Geometry check sheet. Reference: the model listing, model coordinates, mm. A direction names the side the tool comes from. Give positions to 0.01 mm unless a question says otherwise; leave off trailing zeros. Loops run counter-clockwise (first coordinate to the right, second up) from the corner with the lowest first, then second, coordinate; pieces in that order, holes last. Notation, with made-up numbers: (72.5, 32) -> (106.5, 32) arc R26 ccw to (106.5, 70) -> close; hole circle Ø8 at (0.25, 38). An arc over 180 degrees is marked (long way). Answer in a Markdown table with one row per item. Add a question column.
```python
from build123d import *

# Parameters (mm, degrees)
CROQUIS1_W               = 72
CROQUIS1_H               = 74
SALIENTE_EXTRUIR3_DEPTH  = 4
CROQUIS2_W               = 3
CROQUIS2_H               = 6
SALIENTE_EXTRUIR4_DEPTH  = 7.6
CORTAR_EXTRUIR3_DEPTH    = 83.938591741
CROQUIS5_W               = 5
CROQUIS5_H               = 4
SALIENTE_EXTRUIR5_DEPTH  = 1
CROQUIS9_W               = 72
CROQUIS9_H               = 1.5
SALIENTE_EXTRUIR6_DEPTH  = 8
CROQUIS10_W              = 72
CROQUIS10_H              = 5.9
SALIENTE_EXTRUIR7_DEPTH  = 2
CROQUIS11_W              = 10
CROQUIS11_H              = 4.4
SALIENTE_EXTRUIR10_DEPTH = 7
SALIENTE_EXTRUIR14_DEPTH = 10
CROQUIS15_W              = 18
CROQUIS15_H              = 4.4
SALIENTE_EXTRUIR15_DEPTH = 5
CROQUIS16_W              = 72
CROQUIS16_H              = 40
SALIENTE_EXTRUIR16_DEPTH = 10.5
CROQUIS17_W              = 72
CROQUIS17_H              = 5
SALIENTE_EXTRUIR17_DEPTH = 8
CROQUIS18_W              = 72
CROQUIS18_H              = 8
SALIENTE_EXTRUIR19_DEPTH = 2
CROQUIS19_W              = 72
CROQUIS19_H              = 1
CORTAR_EXTRUIR4_DEPTH    = 14.5
CROQUIS20_W              = 72
CROQUIS20_H              = 7
SALIENTE_EXTRUIR20_DEPTH = 65
CROQUIS21_W              = 57
CROQUIS21_H              = 46
CORTAR_EXTRUIR5_DEPTH    = 65


with BuildPart() as part:
    # Croquis1 → Saliente-Extruir3 (new body)
    with BuildSketch(Plane.XY):
        with Locations((0, -2.5)):
            Rectangle(CROQUIS1_W, CROQUIS1_H)
    extrude(amount=SALIENTE_EXTRUIR3_DEPTH)

    # Croquis2 → Saliente-Extruir4 (add)
    with BuildSketch(Plane.XY.offset(4)):
        with Locations((-34.5, -36.5)):
            Rectangle(CROQUIS2_W, CROQUIS2_H)
        with Locations((34.5, -36.5)):
            Rectangle(CROQUIS2_W, CROQUIS2_H)
    extrude(amount=SALIENTE_EXTRUIR4_DEPTH)

    # Croquis3 → Cortar-Extruir3 (cut, through all)
    with BuildSketch(Plane.ZY.offset(36)):
        Polygon((4, -39.5), (11.6, -36.5), (11.6, -39.5), align=None)
    extrude(amount=-CORTAR_EXTRUIR3_DEPTH, mode=Mode.SUBTRACT)

    # Croquis5 → Saliente-Extruir5 (add)
    with BuildSketch(Plane.XY.offset(4)):
        with Locations((-33.5, -30.5)):
            Rectangle(CROQUIS5_W, CROQUIS5_H)
        with Locations((33.5, -29.5)):
            Rectangle(CROQUIS5_W, CROQUIS5_H)
    extrude(amount=SALIENTE_EXTRUIR5_DEPTH)

    # Croquis9 → Saliente-Extruir6 (add)
    with BuildSketch(Plane.XY.offset(4)):
        with Locations((0, -26.35)):
            Rectangle(CROQUIS9_W, CROQUIS9_H)
    extrude(amount=SALIENTE_EXTRUIR6_DEPTH)

    # Croquis10 → Saliente-Extruir7 (add)
    with BuildSketch(Plane.XY.offset(12)):
        with Locations((0, -28.55)):
            Rectangle(CROQUIS10_W, CROQUIS10_H)
    extrude(amount=SALIENTE_EXTRUIR7_DEPTH)

    # Croquis11 → Saliente-Extruir10 (add)
    with BuildSketch(Plane.XY.offset(14)):
        with Locations((-31, -29.3)):
            Rectangle(CROQUIS11_W, CROQUIS11_H)
        with Locations((31, -29.3)):
            Rectangle(CROQUIS11_W, CROQUIS11_H)
    extrude(amount=-SALIENTE_EXTRUIR10_DEPTH)

    # Croquis14 → Saliente-Extruir14 (add)
    with BuildSketch(Plane.XY.offset(4)):
        with BuildLine():
            Line((-9, -23.7), (-9, -25.6))
            Line((-9, -25.6), (-2.1, -25.6))
            ThreePointArc((-2.1, -25.6), (-2.656497116, -24.256497116), (-4, -23.7))
            Line((-4, -23.7), (-9, -23.7))
        make_face()
        with BuildLine():
            Line((-9, -21.2), (-9, -22.2))
            Line((-9, -22.2), (-4, -22.2))
            ThreePointArc((-4, -22.2), (-2.22447191, -22.714955647), (-1, -24.1))
            Line((-1, -24.1), (1, -24.1))
            ThreePointArc((1, -24.1), (2.22447191, -22.714955647), (4, -22.2))
            Line((4, -22.2), (9, -22.2))
            Line((9, -22.2), (9, -21.2))
            Line((9, -21.2), (-9, -21.2))
        make_face()
        with BuildLine():
            ThreePointArc((4, -23.7), (2.656497116, -24.256497116), (2.1, -25.6))
            Line((2.1, -25.6), (9, -25.6))
            Line((9, -25.6), (9, -23.7))
            Line((9, -23.7), (4, -23.7))
        make_face()
    extrude(amount=SALIENTE_EXTRUIR14_DEPTH)

    # Croquis15 → Saliente-Extruir15 (add)
    with BuildSketch(Plane.XY.offset(4)):
        with Locations((0, -23.4)):
            Rectangle(CROQUIS15_W, CROQUIS15_H)
    extrude(amount=SALIENTE_EXTRUIR15_DEPTH)

    # Croquis16 → Saliente-Extruir16 (add)
    with BuildSketch(Plane.XY.offset(4)):
        with Locations((0, 14.5)):
            Rectangle(CROQUIS16_W, CROQUIS16_H)
    extrude(amount=SALIENTE_EXTRUIR16_DEPTH)

    # Croquis17 → Saliente-Extruir17 (add)
    with BuildSketch(Plane.XY.offset(14.5)):
        with Locations((0, 32)):
            Rectangle(CROQUIS17_W, CROQUIS17_H)
    extrude(amount=SALIENTE_EXTRUIR17_DEPTH)

    # Croquis18 → Saliente-Extruir19 (add)
    with BuildSketch(Plane(origin=(0, 34.5, 0), x_dir=(1, 0, 0), z_dir=(0, 1, 0))):
        with Locations((0, -18.5)):
            Rectangle(CROQUIS18_W, CROQUIS18_H)
    extrude(amount=SALIENTE_EXTRUIR19_DEPTH)

    # Croquis19 → Cortar-Extruir4 (cut)
    with BuildSketch(Plane(origin=(0, 0, 0), x_dir=(-1, 0, 0), z_dir=(0, 0, -1))):
        with Locations((0, 34)):
            Rectangle(CROQUIS19_W, CROQUIS19_H)
    extrude(amount=-CORTAR_EXTRUIR4_DEPTH, mode=Mode.SUBTRACT)

    # Croquis20 → Saliente-Extruir20 (add)
    with BuildSketch(Plane(origin=(0, 0, 0), x_dir=(-1, 0, 0), z_dir=(0, 0, -1))):
        with Locations((0, -36)):
            Rectangle(CROQUIS20_W, CROQUIS20_H)
    extrude(amount=SALIENTE_EXTRUIR20_DEPTH)

    # Croquis21 → Cortar-Extruir5 (cut)
    with BuildSketch(Plane(origin=(0, -32.5, 0), x_dir=(1, 0, 0), z_dir=(0, 1, 0))):
        with Locations((2.5, 32)):
            Rectangle(CROQUIS21_W, CROQUIS21_H)
    extrude(amount=-CORTAR_EXTRUIR5_DEPTH, mode=Mode.SUBTRACT)


solid = part.part
```
1. Sectioned sample at C-C (y = -2). Enter the section's corners in (x, z).
2. Sectioned sample at B-B (z = -25). Enter the section's corners in (x, y).
3. Sectioned sample at A-A (x = -19). Enter the section's corners in (y, z).
4. Sectioned sample at D-D (z = -1.5). Enter the section's corners in (x, y), plus the area to 3 significant figures.
5. Release check for a two-part mould opening along Y. For faces 5 (the face through (-1, 33, 22.5)), 6 (the face through (1, 33.5, 7)), 7 (the face through (-23, -25.6, 9)) record: released by +Y, released by -Y, zero draft, split by the parting line, or undercut.
6. Access from +Z, -Z, +X, -X, +Y, -Y to the whole of each face (thin tool, end or side, straight path). Record for faces 1 (the face through (33, -29, 5)), 2 (the face through (26, -29, 10)), 3 (the face through (-1, -5.5, 9)), 4 (the face through (31, -36, -32)).
7. Material ranges on L1, parallel to Z at x = -4.5, y = -33.5; L2, parallel to Z at x = -5.5, y = -28.5; L3, parallel to Y at x = 5.5, z = 5.5, recorded low to high. Write a range as from..to.
8. Gauge pin test, flat ends, axial feed: pin 1 Ø4 at (x, z) = (-14, 17) entering from -Y; pin 2 Ø0.8 at (x, z) = (-33.5, 4.5) entering from +Y; pin 3 Ø5 at (x, y) = (11.5, 20.5) entering from -Z. Record the tip position at first contact, or that the pin passes through.
Response:
| question | item | result |
|---|---|---|
| 1 | outline | (-36, 0) -> (36, 0) -> (36, 14.5) -> (-36, 14.5) -> close |
| 2 | outline | (-36, -39.5) -> (-26, -39.5) -> (-26, -32.5) -> (-36, -32.5) -> close; (31, -39.5) -> (36, -39.5) -> (36, -32.5) -> (31, -32.5) -> close |
| 3 | outline | (-39.5, -65) -> (-32.5, -65) -> (-32.5, -55) -> (-39.5, -55) -> close; (-39.5, -9) -> (-32.5, -9) -> (-32.5, 0) -> (33.5, 0) -> (33.5, 14.5) -> (36.5, 14.5) -> (36.5, 22.5) -> (29.5, 22.5) -> (29.5, 14.5) -> (-5.5, 14.5) -> (-5.5, 4) -> (-25.6, 4) -> (-25.6, 14) -> (-31.5, 14) -> (-31.5, 12) -> (-27.1, 12) -> (-27.1, 4) -> (-39.5, 4) -> close |
| 4 | outline | (-36, -39.5) -> (36, -39.5) -> (36, -32.5) -> (-36, -32.5) -> close |
| 4 | area | 504 mm2 |
| 5 | face 5 | zero draft |
| 5 | face 6 | released by +Y |
| 5 | face 7 | undercut |
| 6 | face 1 | +X, -X |
| 6 | face 2 | -Y |
| 6 | face 3 | +Z, +X, -X |
| 6 | face 4 | +Y, -Y |
| 7 | L1 | z = -65..-55, -9..4 |
| 7 | L2 | z = 0..4, 12..14 |
| 7 | L3 | y = -27.1..-21.2, -5.5..33.5 |
| 8 | pin 1 | stops at y = 29.5 |
| 8 | pin 2 | stops at y = 33.5 |
| 8 | pin 3 | stops at z = 0 |
